Geometry: final body of the model. Coordinates: model frame, mm. A direction names the side the tool comes from. Give positions to 0.01 mm unless a question says otherwise; leave off trailing zeros. Write each loop counter-clockwise with the first axis right and the second up, starting at its lowest first coordinate (ties: lowest second). Pieces come first, ordered by that corner, then holes.
Q1. Pin query (flat end, axial travel): pin 1 (6 mm diameter, centred on y = -2.5, z = 78.5, fed in from -X); pin 2 (4.5 mm diameter, centred on x = -1, z = 7, fed in from -Y); pin 3 (0.8 mm diameter, centred on x = 1, y = 0, fed in from +Z). Return the tip coordinate at first contact, or that it passes through.
Q2. Cut plane B-B on y = 4. Return the cut outline in (x, z).
Q3. Line query: L1, parallel to X at y = 0, z = 84; L2, parallel to Z at x = 8, y = 4; L3, parallel to Y at x = -3, z = 78.5. Output: solid intervals per line, ascending.
Q4. Cut plane D-D on x = 13. Return the cut outline in (y, z), plus the area to 3 significant figures.
Q5. Reachability of faces 5 (the face through (0, -1, 80)), 6 (the face through (5.47, -16.54, 39.93)), 7 (the face through (0, 0.7, 5)) from +Z, -Z, +X, -X, +Y, -Y: full face, straight path, thin tool, end or side. Return the list, or none.
Q6. Cut plane A-A on x = 0. Return the cut outline in (y, z), plus the area to 3 significant figures.
Q7. Draft query along X for faces 1 (the face through (2.86, 0.9, 85.07)), 2 (the face through (17.4, 0.6, 39.9)), 3 (the face through (0, -0.7, 5)), 4 (the face through (0, -1, 0)). Return one class per face: pulls with the +X half, pulls with the -X half, needs draft (parallel to the pull), parting line crosses it, or undercut.
Q8. Cut plane C-C on z = 60. Return the cut outline in (x, y), plus the area to 3 significant figures.
Autodesk Inventor part; units mm, degrees
ref_plane "Work Plane1" through (-14, -11, 93) normal (0, 0, -1) x (0, 1, 0)
ref_plane "YZ Plane" through (0, 0, 0) normal (1, 0, 0) x (0, 1, 0)
ref_plane "XZ Plane" through (0, 0, 0) normal (0, 1, 0) x (-1, 0, 0)
sketch "Sketch1" plane through (0, 0, 0) normal (0, 0, 1) x (1, 0, 0)
  line L0 (2.6, -0.6) -> (-2.6, -0.6)
  line L1 (-2.6, -0.6) -> (-2.6, 0.6)
  line L2 (-2.6, 0.6) -> (2.6, 0.6)
  line L3 (2.6, 0.6) -> (2.6, -0.6)
  circle A0 centre (0, 0) radius 3.6
  line L4 (-2.7, 0.7) -> (-2.7, -0.7)
  line L5 (-2.7, -0.7) -> (2.7, -0.7)
  line L6 (2.7, -0.7) -> (2.7, 0.7)
  line L7 (2.7, 0.7) -> (-2.7, 0.7)
  circle A1 centre (0, 0) radius 5.6
  dimension "d0" = 0.1
  dimension "d5" = 2
extrude "Extrusion1" add sketch "Sketch1" along normal blind 10 contours A0 | A1
sketch "Sketch2" plane through (0, 0, 10) normal (0, 0, 1) x (0, -1, 0)
  line L0 (-0.7, -2.7) -> (-0.7, 2.7)
  line L1 (-0.7, 2.7) -> (0.7, 2.7)
  line L2 (0.7, 2.7) -> (0.7, -2.7)
  line L3 (0.7, -2.7) -> (-0.7, -2.7)
  circle A0 centre (0, 0) radius 3.75
  circle A1 centre (0, 0) radius 5.6
ref_plane "Work Plane1" through (-14, -11, 93) normal (0, 0, -1) x (0, 1, 0)
extrude "Extrusion2" add sketch "Sketch2" along normal blind 80 contours L0 L1 L2 L3 | A0 | A1
ref_plane "Work Plane2" through (14.5169, -8.0562, 35) normal (0, 0, -1) x (-1, 0, 0)
sketch "Sketch4" plane through (0, 0, 90) normal (0, 0, 1) x (1, 0, 0)
  circle A0 centre (0, 0) radius 3
  dimension "d20" = 6
extrude "Extrusion4" cut sketch "Sketch4" against normal blind 10
sketch "Sketch5" plane through (0, 0, 80) normal (0, 0, 1) x (1, 0, 0)
  circle A0 centre (0, 0) radius 3
  circle A1 centre (0, 0) radius 3
  line L0 (-3, 0.5) -> (3, 0.5)
  line L1 (3, 0.5) -> (3, -0.5)
  line L2 (3, -0.5) -> (-3, -0.5)
  line L3 (-3, -0.5) -> (-3, 0.5)
  line L4 (-3, 0.5) -> (3, -0.5) construction
  line L5 (3, 0.5) -> (-3, -0.5) construction
  point P0 (-2.958, -0.5)
  point P1 (2.958, -0.5)
  point P2 (2.958, 0.5)
  point P3 (-2.958, 0.5)
  dimension "d24" = 6
  dimension "d25" = 1
extrude "Extrusion5" add sketch "Sketch5" along normal blind 0.8 contours A0 L2 L0
sketch "Sketch6" plane through (14.5169, -8.0562, 35) normal (0, 0, -1) x (-1, 0, 0)
  circle A0 centre (14.5169, 8.0562) radius 5.6
  circle A1 centre (14.5169, 8.0562) radius 13.6
  line L0 (19.2509, -4.6933) -> (-8.8851, -15.1405)
  line L1 (4.1919, 16.9079) -> (-15.3464, -5.8823)
  line L2 (-8.8851, -15.1405) -> (0.2779, -1.8727)
  line L3 (0.2779, -1.8727) -> (-15.3464, -5.8823)
  line L4 (20.3441, -4.2322) -> (-52.8556, -38.9438)
  line L5 (4.1919, 16.9079) -> (-52.8556, -38.9438)
  arc A2 (-101.4982, -27.3726) -> (-98.3101, -29.4028) centre (-99.5525, -27.8355) ccw
  arc A3 (-98.7514, -19.105) -> (-101.4982, -27.3726) centre (-52.8556, -38.9438) ccw
  line L6 (-98.7514, -19.105) -> (-109.7663, -14.3437)
  arc A4 (-98.2472, 3.2889) -> (-109.7663, -14.3437) centre (-52.8556, -38.9438) ccw
  line L7 (-98.2472, 3.2889) -> (-89.4617, -4.8852)
  arc A5 (-18.7969, -2.3377) -> (-89.4617, -4.8852) centre (-52.8556, -38.9438) ccw
  line L8 (-18.7969, -2.3377) -> (-26.971, -11.1232)
  arc A6 (-41.1368, -75.0917) -> (-26.971, -11.1232) centre (-52.8556, -38.9438) ccw
  line L9 (-41.1368, -75.0917) -> (-42.3055, -71.487)
  arc A7 (-42.3055, -71.487) -> (-59.8761, -67.1138) centre (-52.9931, -76.9436) ccw
  arc A8 (-61.0624, -66.7913) -> (-59.8761, -67.1138) centre (-60.3349, -66.4585) ccw
  arc A9 (-61.0624, -66.7913) -> (-73.0205, -59.8295) centre (-71.9745, -71.7838) ccw
  arc A10 (-73.8866, -58.957) -> (-73.0205, -59.8295) centre (-73.0902, -59.0325) ccw
  arc A11 (-73.8866, -58.957) -> (-80.7617, -46.9489) centre (-85.8331, -57.8246) ccw
  arc A12 (-81.0756, -45.7602) -> (-80.7617, -46.9489) centre (-80.4236, -46.2238) ccw
  arc A13 (-81.0756, -45.7602) -> (-85.3215, -28.1585) centre (-90.8553, -38.8063) ccw
  line L10 (-85.3215, -28.1585) -> (-88.9177, -26.9638)
  arc A14 (-88.9177, -26.9638) -> (-98.3101, -29.4028) centre (-90.8553, -38.8063) ccw
  circle A15 centre (-52.8556, -38.9438) radius 4
  circle A16 centre (-52.8556, -38.9438) radius 18
  circle A17 centre (-52.8556, -38.9438) radius 50
  line L11 (0.2779, -1.8727) -> (-52.8556, -38.9438)
  point P0 (2.5698, 1.558)
  point P1 (4.2932, -0.9124)
  dimension "d30" = 8
  dimension "d34" = 35
  dimension "d36" = 5
  dimension "d37" = 5
  dimension "d39" = 35
extrude "Extrusion6" add sketch "Sketch6" against normal blind 10 contours A1 | A1 L0 L2 L3 L1
fillet "Fillet1" radius 2.5 3 edges at (23.402, -23.1967, 40) (29.8633, -13.9385, 40) (14.2391, -9.9288, 40)
equation "\"d37\" = d36"
equation "\"d39\" = d34"
properties part number "reverser-base"
Data:
1. pin 1: stops at x = -5.6
1. pin 2: stops at y = -5.6
1. pin 3: stops at z = 80.8
2. outline: (-13, 35) - (-3.92, 35) - (-3.92, 0) - (3.92, 0) - (3.92, 35) - (14.48, 35) - (14.48, 45) - (3.92, 45) - (3.92, 90) - (-3.92, 90) - (-3.92, 45) - (-13, 45) - close
3. L1: x = -5.6 to -3, 3 to 5.6
3. L2: z = 35 to 45
3. L3: y = -4.73 to 4.73
4. outline: (-19.33, 35) - (5.73, 35) - (5.73, 45) - (-19.33, 45) - close
4. area: 251 mm2
5. face 5: +Z
5. face 6: +Z, -Z, -X, -Y
5. face 7: -Z
6. outline: (-14.51, 35) - (-5.6, 35) - (-5.6, 0) - (-0.7, 0) - (-0.7, 10) - (0.7, 10) - (0.7, 0) - (5.6, 0) - (5.6, 35) - (13.6, 35) - (13.6, 45) - (5.6, 45) - (5.6, 90) - (3, 90) - (3, 80) - (0.5, 80) - (0.5, 80.8) - (-0.5, 80.8) - (-0.5, 80) - (-3, 80) - (-3, 90) - (-5.6, 90) - (-5.6, 45) - (-14.51, 45) - close
6. area: 1,100 mm2
7. face 1: undercut
7. face 2: pulls with the +X half
7. face 3: undercut
7. face 4: needs draft
8. outline: circle Ø11.2 at (0, 0)
8. area: 98.5 mm2
